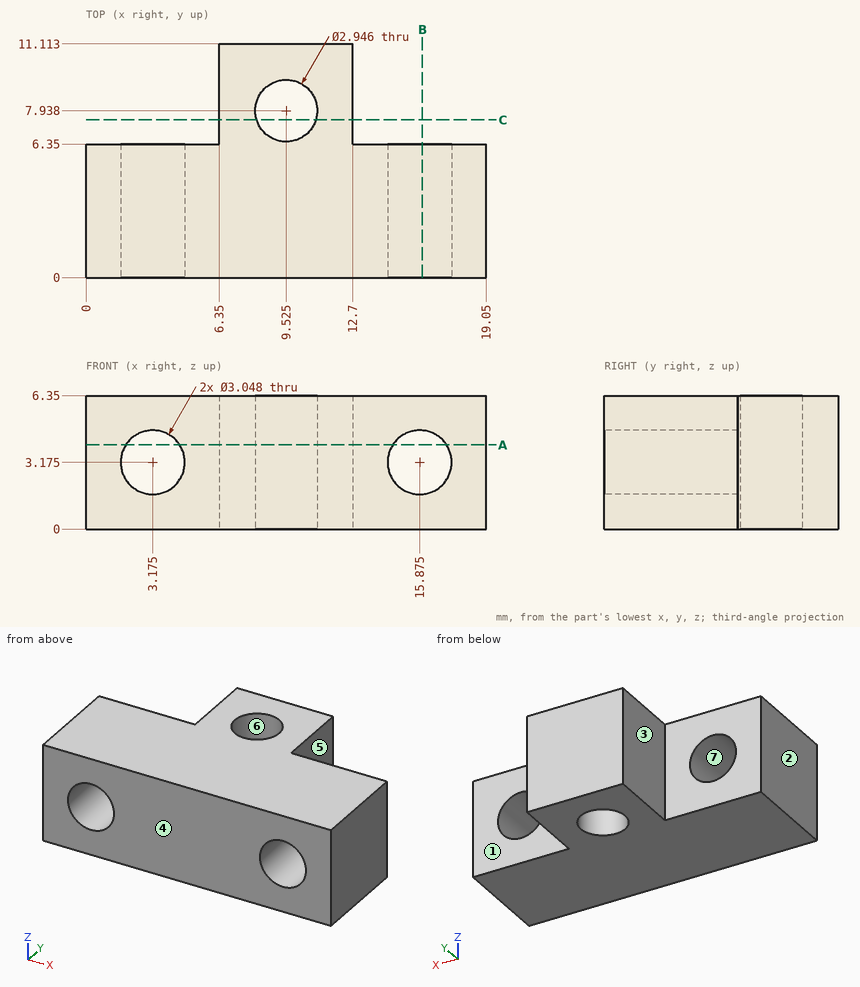
Design review of the part shown in the three views and the two pictorial views. Dimensions are in mm from the part's minimum x, y and z. A direction names the side the tool comes from. Give positions to 0.01 mm unless a question says otherwise; leave off trailing zeros. Loops run counter-clockwise (first coordinate to the right, second up) from the corner with the lowest first, then second, coordinate; pieces in that order, holes last. Notation, with made-up numbers: (-26.5, 54) - (31.5, 54) arc R21 cw to (31.5, 92) - close; hole circle Ø7 at (-37, -20.5). An arc over 180 degrees is marked (long way). Answer as a JSON object with one key per item and string values.
Q1. For the marked faces 1, 2 and 3, list the 3-axis set-ups (+Z, -Z, +X, -X, +Y, -Y) from which the entire face can be reached by the end or side of a thin tool; tool diameter is ignored.
Worked out:
{"face 1": "+Z, -Z, +X, +Y", "face 2": "+Z, -Z, -X, +Y, -Y", "face 3": "+Z, -Z, -X, +Y"}
Q2. Insertion check: pin 1 (1.4 mm diameter, centred on y = 9, z = 2, fed in from +X); pin 2 (3 mm diameter, centred on x = 14.5, z = 2, fed in from +Y). Each pin has a flat end and moves straight along its axis. Give the tip position at first contact, or say it passes through.
Worked out:
{"pin 1": "stops at x = 12.7", "pin 2": "stops at y = 6.35"}
Q3. Mouldability with a two-part tool opening along X and no side actions: class the marked faces 4, 5, 6 and 7 as +X half, -X half, draft (parallel to the pull), parting line (faces both ways), or undercut.
Worked out:
{"face 4": "draft", "face 5": "+X half", "face 6": "undercut", "face 7": "undercut"}
Q4. To check wall thickness, follow line 1 along X through (y, z) = (8, 2.75); line 2 along X through (y, z) = (2.5, 3); line 3 along X through (y, z) = (10.5, 1). State the ranges of each line that lie inside material, in increasing order.
Worked out:
{"line 1": "x = 6.35 to 8.05, 11 to 12.7", "line 2": "x = 0 to 1.66, 4.69 to 14.36, 17.39 to 19.05", "line 3": "x = 6.35 to 12.7"}
Q5. Add section C-C on y = 7.5. State the section outline as (x, z) points.
Worked out:
{"outline": "(6.35, 0) - (8.12, 0) - (8.12, 6.35) - (6.35, 6.35) - close; (10.93, 0) - (12.7, 0) - (12.7, 6.35) - (10.93, 6.35) - close"}
Q6. Add section B-B on x = 16. State the section outline as (y, z) points.
Worked out:
{"outline": "(0, 0) - (6.35, 0) - (6.35, 1.66) - (0, 1.66) - close; (0, 4.69) - (6.35, 4.69) - (6.35, 6.35) - (0, 6.35) - close"}
Q7. Add section A-A on z = 4. Count the separate pieces of the cut face and the enclosed holes in it, plus the area to 3 significant figures.
Worked out:
{"separate pieces": "3", "enclosed holes": "1", "area": "112 mm^2"}
